Verification items for the finished model (mm, model axes). A direction names the side the tool comes from. Round coordinates to 2 decimals unless told otherwise and drop trailing zeros. Write each loop counter-clockwise with the first axis right and the second up, starting at its lowest first coordinate (ties: lowest second). Pieces come first, ordered by that corner, then holes. Notation, with made-up numbers: M 27.5,-38.5 L 45.5,-38.5 A34 ccw 45.5,-2.5 Z; hole C 73.5,18 d11. An arc over 180 degrees is marked long. Answer in a Markdown table with one row per item. Add a question column.
1. Sectioned sample at C-C on x = 0. Record the cut outline in (y, z), plus the area to 4 significant figures.
2. Sectioned sample at A-A on x = 13. Record the cut outline in (y, z), plus the area to 3 significant figures.
3. Sectioned sample at D-D on y = 10. Record the cut outline in (x, z), plus the area to 3 significant figures.
4. Material ranges on probe 1 along Y at (x, z) = (4, 1.65); probe 2 along Y at (x, z) = (-13.5, 0.2); probe 3 along Y at (x, z) = (-8.5, 0.4), recorded low to high.
5. Sectioned sample at B-B on y = -9.5. Record the cut outline in (x, z).
6. Set-up check for faces 4 (the flat face through (-7.5, -8.6, 0.5)), 5 (the flat face through (10.4, -3, 2)): record each of +Z, -Z, +X, -X, +Y, -Y from which the full face is reachable in a straight line by a thin tool's end or side.
7. Draft check along X on faces 1 (the flat face through (-0.3, 0.3, 0)), 2 (the flat face through (-19, 0, 1)), 3 (the flat face through (9.65, 0.6, 0.5)). Enter one of: pulls with the +X half, pulls with the -X half, needs draft (parallel to the pull), parting line crosses it, or undercut.
```python
from build123d import *

# Parameters (mm, degrees)
SKETCH_W        = 38
SKETCH_H        = 36
PAD_DEPTH       = 2.5
SKETCH001_W     = 14
SKETCH001_H     = 14
POCKET_DEPTH    = 1.4
SKETCH002_W     = 15
SKETCH002_H     = 14
POCKET001_DEPTH = 1.1


with BuildPart() as part:
    # Sketch → Pad (new body)
    with BuildSketch(Plane.XY):
        Rectangle(SKETCH_W, SKETCH_H)
    extrude(amount=PAD_DEPTH)

    # Sketch001 (on DatumPlane) → Pocket (cut)
    with BuildSketch(Plane.XY.offset(2.5)):
        with Locations((-9, 8.5)):
            Rectangle(SKETCH001_W, SKETCH001_H)
        with Locations((9, 8.5)):
            Rectangle(SKETCH001_W, SKETCH001_H)
        with Locations((0, -8.5)):
            Rectangle(SKETCH001_W, SKETCH001_H)
        Polygon((10.4, -0.9), (10.4, -4.4), (8.9, -4.4), (8.9, -11.4), (15.4, -11.4), (15.4, -4.4), (13.9, -4.4), (13.9, -0.9), align=None)
        Polygon((-15.4, -11.4), (-8.9, -11.4), (-8.9, -4.4), (-10.4, -4.4), (-10.4, -0.9), (-13.9, -0.9), (-13.9, -4.4), (-15.4, -4.4), align=None)
    extrude(amount=-POCKET_DEPTH, mode=Mode.SUBTRACT)

    # Sketch002 → Pocket001 (cut)
    with BuildSketch(Plane.XY):
        with Locations((9, 8.5)):
            Rectangle(SKETCH002_W, SKETCH002_H)
        with Locations((-9, 8.5)):
            Rectangle(SKETCH002_W, SKETCH002_H)
        with Locations((0, -8.5)):
            Rectangle(SKETCH002_W, SKETCH002_H)
        Polygon((8.15, -11.9), (8.15, -3.9), (9.65, -3.9), (9.65, -1.4), (-9.65, -1.4), (-9.65, -3.9), (-8.15, -3.9), (-8.15, -11.9), (-16.15, -11.9), (-16.15, -3.9), (-14.65, -3.9), (-14.65, 1.1), (-9.65, 1.1), (-9.65, 0.1), (9.65, 0.1), (9.65, 1.1), (14.65, 1.1), (14.65, -3.9), (16.15, -3.9), (16.15, -11.9), align=None)
    extrude(amount=POCKET001_DEPTH, mode=Mode.SUBTRACT)


solid = part.part
```
Geometry check:
| question | item | result |
|---|---|---|
| 1 | outline | M -18,0 L -15.5,0 L -15.5,2.5 L -18,2.5 Z; M -1.5,0 L -1.4,0 L -1.4,1.1 L 0.1,1.1 L 0.1,0 L 18,0 L 18,2.5 L -1.5,2.5 Z |
| 1 | area | 53.35 mm2 |
| 2 | outline | M -18,0 L -11.9,0 L -11.9,1.1 L -11.4,1.1 L -11.4,2.5 L -18,2.5 Z; M -0.9,1.1 L 1.1,1.1 L 1.1,0 L 1.5,0 L 1.5,2.5 L -0.9,2.5 Z; M 15.5,0 L 18,0 L 18,2.5 L 15.5,2.5 Z |
| 2 | area | 26.0 mm2 |
| 3 | outline | M -19,0 L -16.5,0 L -16.5,1.1 L -16,1.1 L -16,2.5 L -19,2.5 Z; M -2,1.1 L -1.5,1.1 L -1.5,0 L 1.5,0 L 1.5,1.1 L 2,1.1 L 2,2.5 L -2,2.5 Z; M 16,1.1 L 16.5,1.1 L 16.5,0 L 19,0 L 19,2.5 L 16,2.5 Z |
| 3 | area | 22.8 mm2 |
| 4 | probe 1 | y = -18 to -15.5, -1.5 to 1.5, 15.5 to 18 |
| 4 | probe 2 | y = -18 to -11.9, 1.1 to 1.5, 15.5 to 18 |
| 4 | probe 3 | y = -18 to -11.9, -3.9 to -1.4, 0.1 to 1.5, 15.5 to 18 |
| 5 | outline | M -19,0 L -16.15,0 L -16.15,1.1 L -15.4,1.1 L -15.4,2.5 L -19,2.5 Z; M -8.9,1.1 L -8.15,1.1 L -8.15,0 L -7.5,0 L -7.5,1.1 L -7,1.1 L -7,2.5 L -8.9,2.5 Z; M 7,1.1 L 7.5,1.1 L 7.5,0 L 8.15,0 L 8.15,1.1 L 8.9,1.1 L 8.9,2.5 L 7,2.5 Z; M 15.4,1.1 L 16.15,1.1 L 16.15,0 L 19,0 L 19,2.5 L 15.4,2.5 Z |
| 6 | face 4 | -Z |
| 6 | face 5 | +Z, -Z |
| 7 | face 1 | needs draft |
| 7 | face 2 | pulls with the -X half |
| 7 | face 3 | undercut |
